Can you work these out from the drawing? Everything is in mm from the part's minimum corner. Coordinates: 2 decimals unless noted, no trailing zeros. Loops run counter-clockwise (first coordinate to the right, second up) from the corner with the lowest first, then second, coordinate; pieces in that order, holes last. Notation, with made-up numbers: (49.25, 55) - (92.25, 55) arc R36 ccw to (92.25, 92) - close; hole circle Ø5 at (70.5, 61). An arc over 180 degrees is marked (long way). Use CSV: the item, a comma, the result in double quotes.
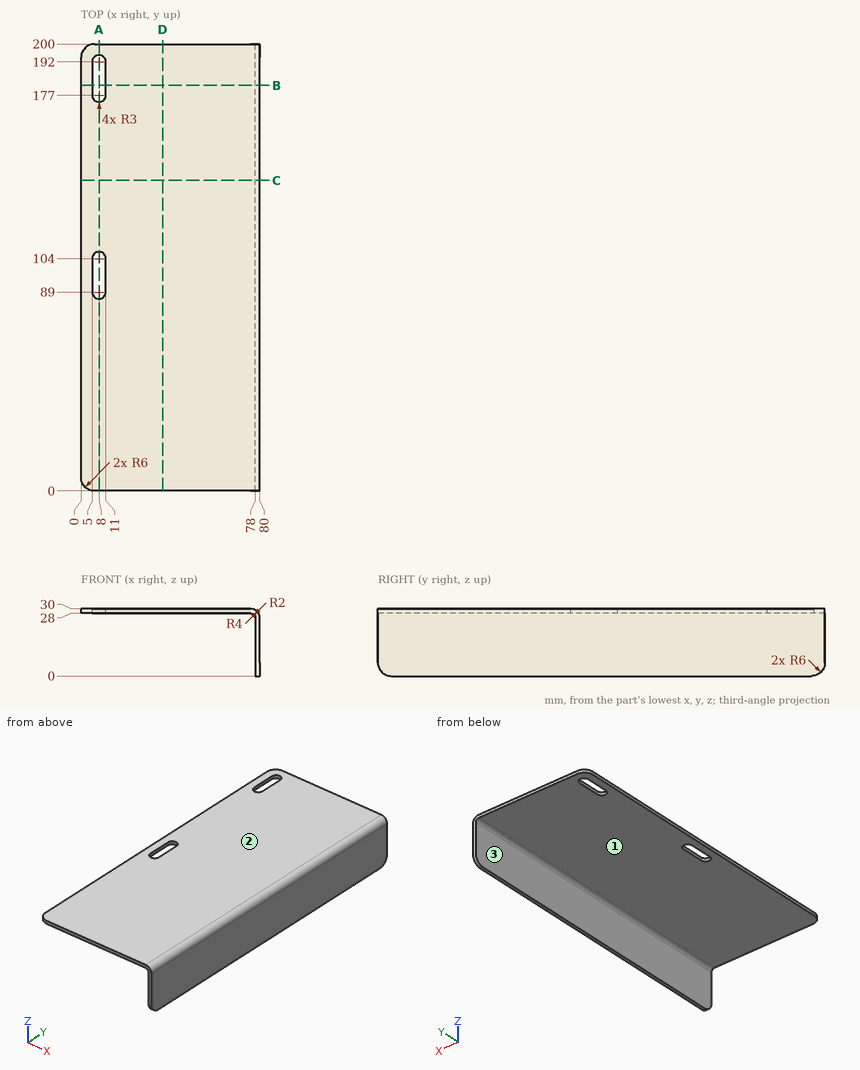
(1) Suppose I cut it at A-A (x = 8). Write out the boundary of the cut face in (y, z), plus the area to 3 significant figures.
Computed:
outline,"(0, 28) - (86, 28) - (86, 30) - (0, 30) - close; (107, 28) - (174, 28) - (174, 30) - (107, 30) - close; (195, 28) - (200, 28) - (200, 30) - (195, 30) - close"
area,"316 mm²"
(2) Thinking about a two-plate mould opening in Z: for the marked faces 1, 2 and 3, which applies, +Z half, -Z half, draft (parallel to the pull), parting line (faces both ways), or undercut?
Computed:
face 1,"-Z half"
face 2,"+Z half"
face 3,"draft"
(3) Suppose I cut it at C-C (y = 139). Write out the boundary of the cut face in (x, z).
Computed:
outline,"(0, 28) - (76, 28) arc R2 cw to (78, 26) - (78, 0) - (80, 0) - (80, 26) arc R4 ccw to (76, 30) - (0, 30) - close"
(4) Please list where these lines run through material, in increasing order: line 1 (Z direction, x = 9, y = 153); line 2 (X direction, y = 100, z = 13.25); line 3 (X direction, y = 23, z = 28.25).
Computed:
line 1,"z = 28 to 30"
line 2,"x = 78 to 80"
line 3,"x = 0 to 79.31"
(5) Will these pins go through, and if not, where does the flat tip stop? pin 1 (1 mm diameter, centred on x = 46.5, y = 63.5, fed in from -Z); pin 2 (13 mm diameter, centred on y = 107.5, z = 17, fed in from -X); pin 3 (1.6 mm diameter, centred on y = 96, z = 29, fed in from +X).
Computed:
pin 1,"stops at z = 28"
pin 2,"stops at x = 78"
pin 3,"stops at x = 79.34"
(6) Suppose I cut it at D-D (x = 36.5). Write out the boundary of the cut face in (y, z).
Computed:
outline,"(0, 28) - (200, 28) - (200, 30) - (0, 30) - close"
(7) Suppose I cut it at B-B (y = 181.5). Write out the boundary of the cut face in (x, z).
Computed:
outline,"(0, 28) - (5, 28) - (5, 30) - (0, 30) - close; (11, 28) - (76, 28) arc R2 cw to (78, 26) - (78, 0) - (80, 0) - (80, 26) arc R4 ccw to (76, 30) - (11, 30) - close"
